Can you work these out from the model? Positions are in its coordinate system, mm. A direction names the side the tool comes from. Coordinates: 2 decimals unless noted, no trailing zeros. Order: outer loops, then holes, each group sorted by start corner. A loop starts at its lowest first (then second) coordinate and runs counter-clockwise, first axis right, second up. Notation, with made-up numbers: (76.5, 83) -> (92.5, 83) arc R22 cw to (92.5, 122) -> close; hole circle Ø10 at (-11.75, 71). An arc over 180 degrees is marked (long way). Answer as a JSON object with one key per item and string values. Group by question number.
(1) I want a section at C-C, the plane y = 0. List the corners of the cut face in (x, z) for me.
(2) I want a section at A-A, the plane z = -23. List the corners of the cut face in (x, y) for me, plus the area to 3 significant figures.
(3) If we mould it in two halves opening along Y, with no side actions, what happens to faces 4 (the cylindrical face through (34, 0, 8)), 5 (the flat face through (24.002, -31.824, -3.944)), 6 (the flat face through (0, 0, 32))? For each: pulls with the +Y half, pulls with the -Y half, needs draft (parallel to the pull), parting line crosses it, or undercut.
(4) I want a section at D-D, the plane x = 0. List the corners of the cut face in (y, z) for me, plus the area to 3 significant figures.
(5) I want a section at B-B, the plane z = -5. State how many separate pieces and enclosed holes the cut face has, plus the area to 3 significant figures.
(6) Which directions (+Z, -Z, +X, -X, +Y, -Y) give clear straight access to the entire face, cutting with the end or side of a thin tool? Please do faces 1 (the flat face through (-36, -22, -19)), 2 (the flat face through (-36, -24, 0)), 3 (the flat face through (-32.92, 24.4, -3.94)).
(7) For pin 1 (3 mm diameter, centred on x = -52, y = -4, fed in from -Z); pin 2 (2.5 mm diameter, centred on x = 22, y = -30.5, fed in from +Z); pin 3 (1.6 mm diameter, centred on x = -35, y = -25, fed in from -Z); pin 4 (12 mm diameter, centred on x = 11, z = -17, fed in from -Y), each with a flat end and sliding along its axis, tell me the tip position at first contact or that it passes through.
(8) I need wall thicknesses on line 1 (Z direction, x = -20.5, y = 2.5); line 2 (Y direction, x = 22, z = -1); line 3 (X direction, y = -25, z = 1.75). Which ranges of each line are inside material? Lowest first, please.
from build123d import *

# Parameters (mm, degrees)
ESQUISSE1_R             = 1.6
BOSS_EXTRU_1_DEPTH      = 10
ESQUISSE2_R             = 32.8
BOSS_EXTRU_2_DEPTH      = 22
ENL_V_MAT_EXTRU_1_DEPTH = 3.5
BOSS_EXTRU_3_REACH      = 12
ESQUISSE4_R             = 32.8
ESQUISSE5_R             = 16
BOSS_EXTRU_4_DEPTH      = 19
ESQUISSE6_R             = 1
BOSS_EXTRU_5_DEPTH      = 27
BOSS_EXTRU_6_DEPTH      = 1.5
ESQUISSE8_R             = 5
BOSS_EXTRU_7_DEPTH      = 5.5
SKETCH2_R               = 4
SKETCH2_R_2             = 3
BOSS_EXTRUDE1_DEPTH     = 9.5


with BuildPart() as part:
    # Esquisse1 → Boss.-Extru.1 (new body)
    with BuildSketch(Plane.XY):
        with BuildLine():
            ThreePointArc((-56.3, -16.861494596), (-60.528670487, -14.599558136), (-64.01, -11.301322931))
            ThreePointArc((-64.01, -11.301322931), (-65, 0), (-64.01, 11.301322931))
            ThreePointArc((-64.01, 11.301322931), (-60.528670487, 14.599558136), (-56.3, 16.861494596))
            Line((-56.3, 16.861494596), (-39.624688626, 23.091930519))
            ThreePointArc((-39.624688626, 23.091930519), (-36.690940127, 29.525679018), (-30.257191628, 26.591930519))
            Line((-30.257191628, 26.591930519), (-12.425, 33.254614341))
            ThreePointArc((-12.425, 33.254614341), (1.381675102, 35.473102119), (14.973963383, 32.187426436))
            Line((14.973963383, 32.187426436), (20.756023105, 34.801647207))
            ThreePointArc((20.756023105, 34.801647207), (24.347774736, 34.238511045), (26, 31))
            Line((26, 31), (25.359978077, 24.841930519))
            ThreePointArc((25.359978077, 24.841930519), (35.5, 0), (25.359978077, -24.841930519))
            Line((25.359978077, -24.841930519), (26, -31))
            ThreePointArc((26, -31), (24.347774736, -34.238511045), (20.756023105, -34.801647207))
            Line((20.756023105, -34.801647207), (14.973963383, -32.187426436))
            ThreePointArc((14.973963383, -32.187426436), (1.381675102, -35.473102119), (-12.425, -33.254614341))
            Line((-12.425, -33.254614341), (-30.257191628, -26.591930519))
            ThreePointArc((-30.257191628, -26.591930519), (-36.690940127, -29.525679018), (-39.624688626, -23.091930519))
            Line((-39.624688626, -23.091930519), (-56.3, -16.861494596))
        make_face()
        with Locations((-35, -25)):
            Circle(ESQUISSE1_R, mode=Mode.SUBTRACT)
        with Locations((22, 31)):
            Circle(ESQUISSE1_R, mode=Mode.SUBTRACT)
        with Locations((-35, 25)):
            Circle(ESQUISSE1_R, mode=Mode.SUBTRACT)
        with Locations((22, -31)):
            Circle(ESQUISSE1_R, mode=Mode.SUBTRACT)
    extrude(amount=BOSS_EXTRU_1_DEPTH)

    # Esquisse2 → Boss.-Extru.2 (add)
    with BuildSketch(Plane.XY.offset(10)):
        Circle(ESQUISSE2_R)
    extrude(amount=BOSS_EXTRU_2_DEPTH)

    # Esquisse3 → Enlèv. mat.-Extru.1 (cut)
    with BuildSketch(Plane.XY.offset(10)):
        with BuildLine():
            Line((-55.775, -15.456370046), (-37.378202776, -22.330008789))
            ThreePointArc((-37.378202776, -22.330008789), (-36.165940127, -28.120554469), (-31.453677478, -24.543603151))
            Line((-31.453677478, -24.543603151), (-11.9, -31.849489792))
            ThreePointArc((-11.9, -31.849489792), (1.664031028, -33.959255009), (14.956816294, -30.533484019))
            Line((14.956816294, -30.533484019), (21.291141631, -33.397398551))
            ThreePointArc((21.291141631, -33.397398551), (23.468656713, -33.023128137), (24.499056843, -31.06866508))
            Line((24.499056843, -31.06866508), (23.79417774, -24.286562245))
            ThreePointArc((23.79417774, -24.286562245), (34, 0), (23.79417774, 24.286562245))
            Line((23.79417774, 24.286562245), (24.499056843, 31.06866508))
            ThreePointArc((24.499056843, 31.06866508), (23.468656713, 33.023128137), (21.291141631, 33.397398551))
            Line((21.291141631, 33.397398551), (14.956816294, 30.533484019))
            ThreePointArc((14.956816294, 30.533484019), (1.664031028, 33.959255009), (-11.9, 31.849489792))
            Line((-11.9, 31.849489792), (-31.453677478, 24.543603151))
            ThreePointArc((-31.453677478, 24.543603151), (-36.165940127, 28.120554469), (-37.378202776, 22.330008789))
            Line((-37.378202776, 22.330008789), (-55.775, 15.456370046))
            ThreePointArc((-55.775, 15.456370046), (-59.496201473, 13.493411636), (-62.6, 10.653168543))
            ThreePointArc((-62.6, 10.653168543), (-63.5, 0), (-62.6, -10.653168543))
            ThreePointArc((-62.6, -10.653168543), (-59.496201473, -13.493411636), (-55.775, -15.456370046))
        make_face()
    extrude(amount=-ENL_V_MAT_EXTRU_1_DEPTH, mode=Mode.SUBTRACT)

    # Esquisse4 → Boss.-Extru.3 (add, up to next)
    with BuildSketch(Plane(origin=(0, 0, 10), x_dir=(-1, 0, 0), z_dir=(0, 0, -1)), mode=Mode.PRIVATE) as boss_extru_3_sk1:
        Circle(ESQUISSE4_R)
    boss_extru_3_tool1 = extrude(boss_extru_3_sk1.sketch, amount=BOSS_EXTRU_3_REACH, mode=Mode.PRIVATE) - part.part
    add(boss_extru_3_tool1.solids().sort_by_distance((0, 0, 10))[0])

    # Esquisse5 → Boss.-Extru.4 (add)
    with BuildSketch(Plane(origin=(0, 0, 0), x_dir=(-1, 0, 0), z_dir=(0, 0, -1))):
        with Locations((50, 0)):
            Circle(ESQUISSE5_R)
    extrude(amount=BOSS_EXTRU_4_DEPTH)

    # Esquisse6 → Boss.-Extru.5 (add)
    with BuildSketch(Plane(origin=(0, 0, 0), x_dir=(-1, 0, 0), z_dir=(0, 0, -1))):
        Polygon((-20.489225606, -29.008126327), (-22.969626005, -28.695694159), (-24.480400399, -30.687567832), (-23.510774394, -32.991873673), (-21.030373995, -33.304305841), (-19.519599601, -31.312432168), align=None)
        with Locations((-22, -31)):
            Circle(ESQUISSE6_R, mode=Mode.SUBTRACT)
        Polygon((36.086835018, -22.748602735), (33.593650283, -22.933074633), (32.506815266, -25.184471898), (33.913164982, -27.251397265), (36.406349717, -27.066925367), (37.493184734, -24.815528102), align=None)
        with Locations((35, -25)):
            Circle(ESQUISSE6_R, mode=Mode.SUBTRACT)
        Polygon((36.720274889, 26.814016072), (34.289153443, 27.396809791), (32.568878555, 25.582793719), (33.279725111, 23.185983928), (35.710846557, 22.603190209), (37.431121445, 24.417206281), align=None)
        with Locations((35, 25)):
            Circle(ESQUISSE6_R, mode=Mode.SUBTRACT)
        Polygon((-19.952160425, 32.43399898), (-22.217959758, 33.490480585), (-24.265799333, 32.056481605), (-24.047839575, 29.56600102), (-21.782040242, 28.509519415), (-19.734200667, 29.943518395), align=None)
        with Locations((-22, 31)):
            Circle(ESQUISSE6_R, mode=Mode.SUBTRACT)
    extrude(amount=BOSS_EXTRU_5_DEPTH)

    # Esquisse7 → Boss.-Extru.6 (add)
    with BuildSketch(Plane(origin=(0, 0, -8), x_dir=(-1, 0, 0), z_dir=(0, 0, -1))):
        with BuildLine():
            Line((30.257191628, 26.591930519), (12.425, 33.254614341))
            ThreePointArc((12.425, 33.254614341), (-1.381675102, 35.473102119), (-14.973963383, 32.187426436))
            Line((-14.973963383, 32.187426436), (-20.756023105, 34.801647207))
            ThreePointArc((-20.756023105, 34.801647207), (-24.347774736, 34.238511045), (-26, 31))
            Line((-26, 31), (-25.359978077, 24.841930519))
            ThreePointArc((-25.359978077, 24.841930519), (-35.5, 0), (-25.359978077, -24.841930519))
            Line((-25.359978077, -24.841930519), (-26, -31))
            ThreePointArc((-26, -31), (-24.347774736, -34.238511045), (-20.756023105, -34.801647207))
            Line((-20.756023105, -34.801647207), (-14.973963383, -32.187426436))
            ThreePointArc((-14.973963383, -32.187426436), (-1.381675102, -35.473102119), (12.425, -33.254614341))
            Line((12.425, -33.254614341), (30.257191628, -26.591930519))
            ThreePointArc((30.257191628, -26.591930519), (36.690940127, -29.525679018), (39.624688626, -23.091930519))
            ThreePointArc((39.624688626, -23.091930519), (33.487603548, 0), (39.624688626, 23.091930519))
            ThreePointArc((39.624688626, 23.091930519), (36.690940127, 29.525679018), (30.257191628, 26.591930519))
        make_face()
    extrude(amount=BOSS_EXTRU_6_DEPTH)

    # Esquisse8 → Boss.-Extru.7 (add)
    with BuildSketch(Plane.XY.offset(6.5)):
        with Locations((-50, 0)):
            Circle(ESQUISSE8_R)
    extrude(amount=BOSS_EXTRU_7_DEPTH)

    # Sketch2 → Boss-Extrude1 (add)
    with BuildSketch(Plane(origin=(0, 0, -9.5), x_dir=(-1, 0, 0), z_dir=(0, 0, -1))):
        with Locations((-22, 31)):
            Circle(SKETCH2_R)
        with Locations((-22, 31)):
            Circle(SKETCH2_R_2, mode=Mode.SUBTRACT)
        with Locations((35, 25)):
            Circle(SKETCH2_R)
        with Locations((35, 25)):
            Circle(SKETCH2_R_2, mode=Mode.SUBTRACT)
        with Locations((-22, -31)):
            Circle(SKETCH2_R)
        with Locations((-22, -31)):
            Circle(SKETCH2_R_2, mode=Mode.SUBTRACT)
        with Locations((35, -25)):
            Circle(SKETCH2_R)
        with Locations((35, -25)):
            Circle(SKETCH2_R_2, mode=Mode.SUBTRACT)
    extrude(amount=BOSS_EXTRUDE1_DEPTH)


solid = part.part
Computed values:
{
 "1": {"outline": "(-66, -19) -> (-34, -19) -> (-34, 0) -> (35.5, 0) -> (35.5, 10) -> (34, 10) -> (34, 6.5) -> (32.8, 6.5) -> (32.8, 32) -> (-32.8, 32) -> (-32.8, 6.5) -> (-45, 6.5) -> (-45, 12) -> (-55, 12) -> (-55, 6.5) -> (-63.5, 6.5) -> (-63.5, 10) -> (-65, 10) -> (-65, 0) -> (-66, 0) -> close; (-33.49, -9.5) -> (35.5, -9.5) -> (35.5, -8) -> (-33.49, -8) -> close"},
 "2": {"outline": "(-37.49, -24.82) -> (-36.41, -27.07) -> (-33.91, -27.25) -> (-32.51, -25.18) -> (-33.59, -22.93) -> (-36.09, -22.75) -> close; (-37.43, 24.42) -> (-35.71, 22.6) -> (-33.28, 23.19) -> (-32.57, 25.58) -> (-34.29, 27.4) -> (-36.72, 26.81) -> close; (19.52, -31.31) -> (21.03, -33.3) -> (23.51, -32.99) -> (24.48, -30.69) -> (22.97, -28.7) -> (20.49, -29.01) -> close; (19.73, 29.94) -> (21.78, 28.51) -> (24.05, 29.57) -> (24.27, 32.06) -> (22.22, 33.49) -> (19.95, 32.43) -> close; hole circle Ø2 at (-35, -25); hole circle Ø2 at (-35, 25); hole circle Ø2 at (22, -31); hole circle Ø2 at (22, 31)", "area": "52.4 mm2"},
 "3": {"face 4": "undercut", "face 5": "pulls with the -Y half", "face 6": "needs draft"},
 "4": {"outline": "(-35.5, -9.5) -> (35.5, -9.5) -> (35.5, -8) -> (-35.5, -8) -> close; (-35.5, 0) -> (35.5, 0) -> (35.5, 10) -> (34, 10) -> (34, 6.5) -> (32.8, 6.5) -> (32.8, 32) -> (-32.8, 32) -> (-32.8, 6.5) -> (-34, 6.5) -> (-34, 10) -> (-35.5, 10) -> close", "area": "2,250 mm2"},
 "5": {"separate pieces": "5", "enclosed holes": "4", "area": "857 mm2"},
 "6": {"face 1": "-Z", "face 2": "+Z", "face 3": "+X"},
 "7": {"pin 1": "stops at z = -19", "pin 2": "stops at z = 6.5", "pin 3": "stops at z = -9.5", "pin 4": "passes through"},
 "8": {"line 1": "z = -9.5 to -8, 0 to 32", "line 2": "y = -33.18 to -32, -30 to -28.82, 28.61 to 30, 32 to 33.39", "line 3": "x = -39.94 to -36.6, -33.4 to 25.38"}
}
